Could you check a few things on this drawing? It's one solid part, dimensions in mm from its lowest x, y, z. Coordinates: 2 decimals unless noted, no trailing zeros. Order: outer loops, then holes, each group sorted by start corner. A loop starts at its lowest first (then second) coordinate and runs counter-clockwise, first axis right, second up.
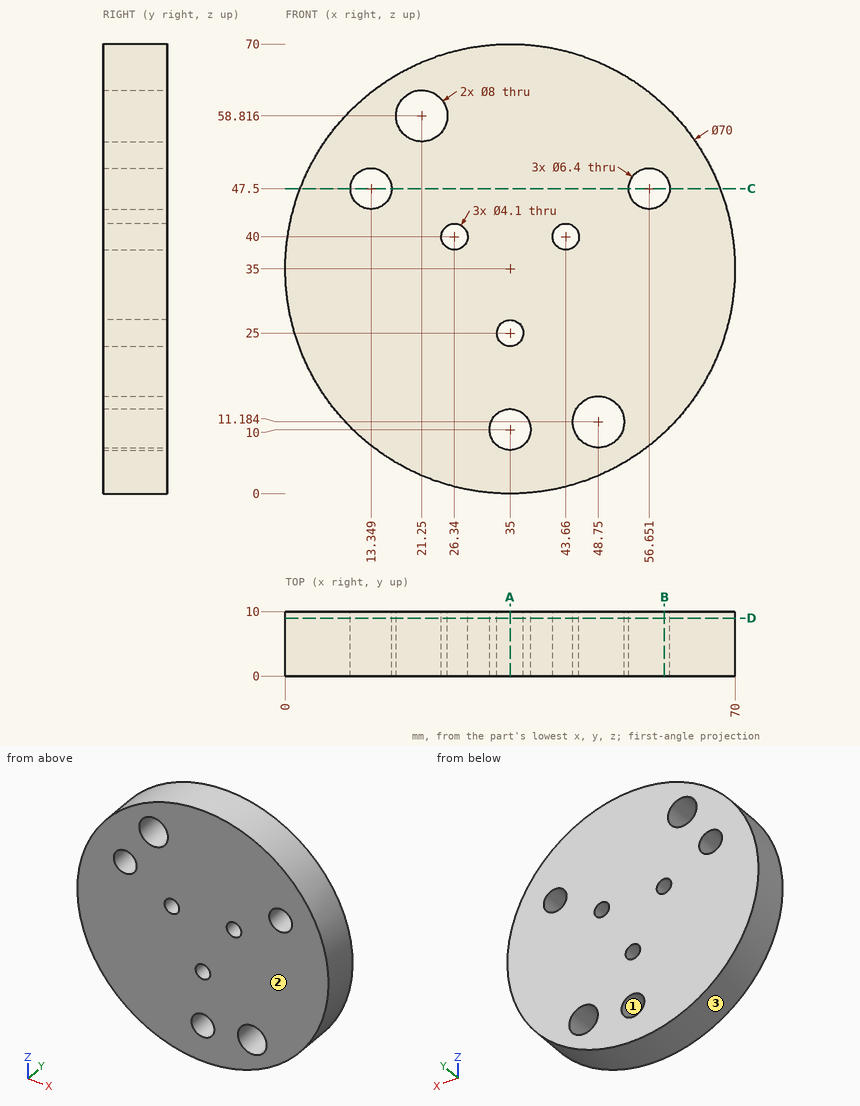
1. Imagine slicing it at A-A on x = 35. Please give me the cut outline in (y, z).
Completed:
outline: (0, 0) - (10, 0) - (10, 6.8) - (0, 6.8) - close; (0, 13.2) - (10, 13.2) - (10, 22.95) - (0, 22.95) - close; (0, 27.05) - (10, 27.05) - (10, 70) - (0, 70) - close
2. Please list where these lines run through material, in increasing order: probe 1 along X at (y, z) = (4.25, 40); probe 2 along X at (y, z) = (3.75, 47.5); probe 3 along Z at (x, y) = (55.5, 4) (1 decimal).
Completed:
probe 1: x = 0.36 to 24.29, 28.39 to 41.61, 45.71 to 69.64
probe 2: x = 2.31 to 10.15, 16.55 to 53.45, 59.85 to 67.69
probe 3: z = 6.6 to 44.5, 50.5 to 63.4
3. Thinking about a two-plate mould opening in X: for the marked faces 1, 2 and 3, which applies, pulls with the +X half, pulls with the -X half, needs draft (parallel to the pull), parting line crosses it, or undercut?
Completed:
face 1: undercut
face 2: needs draft
face 3: parting line crosses it
4. I'm going to push flat-ended pins straight in: pin 1 (2 mm diameter, centred on x = 48, y = 5.5, fed in from -Z); pin 2 (7 mm diameter, centred on x = 48.75, z = 11.18, fed in from -Y); pin 3 (3 mm diameter, centred on y = 4.5, z = 49, fed in from -X); pin 4 (1.5 mm diameter, centred on x = 50, y = 8, fed in from -Z). Where does each tip first touch, or does it pass through?
Completed:
pin 1: stops at z = 2.12
pin 2: passes through
pin 3: stops at x = 2.31
pin 4: stops at z = 3.03
5. Imagine slicing it at D-D on y = 9. Give the number of separate pieces and of enclosed holes in the cut face, then the cut area to 3 significant figures.
Completed:
separate pieces: 1
enclosed holes: 8
area: 3,610 mm2
6. Imagine slicing it at C-C on z = 47.5. Please give me the cut outline in (x, y), then the cut area to 3 significant figures.
Completed:
outline: (2.31, 0) - (10.15, 0) - (10.15, 10) - (2.31, 10) - close; (16.55, 0) - (53.45, 0) - (53.45, 10) - (16.55, 10) - close; (59.85, 0) - (67.69, 0) - (67.69, 10) - (59.85, 10) - close
area: 526 mm2
7. Imagine slicing it at B-B on x = 59. Please give me the cut outline in (y, z) (1 decimal).
Completed:
outline: (0, 9.5) - (10, 9.5) - (10, 45.3) - (0, 45.3) - close; (0, 49.7) - (10, 49.7) - (10, 60.5) - (0, 60.5) - close
